Work out the finished part from the listing and answer in its coordinate system (mm). Give positions to 0.01 mm unless a question says otherwise; leave off trailing zeros. Loops run counter-clockwise (first coordinate to the right, second up) from the corner with the lowest first, then second, coordinate; pieces in that order, holes last. Notation, with made-up numbers: (31, -11) - (82, -11) arc R16 ccw to (82, -1) - close; hole circle Ø10 at (55, -8.5). An arc over 180 degrees is marked (long way). Use one line per item in the form item = value. Start each with the question number.
from build123d import *

# Parameters (mm, degrees)
BOSS_EXTRUDE1_DEPTH = 10
SKETCH2_R           = 1
CUT_EXTRUDE1_DEPTH  = 11.599213807
CHAMFER2_SIZE       = 1
FILLET1_R           = 0.5


with BuildPart() as part:
    # Sketch1 → Boss-Extrude1 (new body)
    with BuildSketch(Plane(origin=(0, 0, 0), x_dir=(1, 0, 0), z_dir=(0, 1, 0))):
        Polygon((0, 2.655811238), (-2.3, 1.327905619), (-2.3, -1.327905619), (0, -2.655811238), (2.3, -1.327905619), (2.3, 1.327905619), align=None)
    extrude(amount=BOSS_EXTRUDE1_DEPTH)

    # Sketch2 → Cut-Extrude1 (cut, through all)
    with BuildSketch(Plane(origin=(0, 10, 0), x_dir=(1, 0, 0), z_dir=(0, 1, 0))):
        with Locations(Location((0, 0, 0), (0, 0, 270))):
            Circle(SKETCH2_R)
    extrude(amount=-CUT_EXTRUDE1_DEPTH, mode=Mode.SUBTRACT)

    # Chamfer2
    chamfer2_edges = [part.edges().sort_by_distance(p)[0] for p in [
        (0, 0, -1),
        (0, 10, -1),
    ]]
    chamfer(chamfer2_edges, length=CHAMFER2_SIZE)

    # Fillet1
    fillet1_edges = [part.edges().sort_by_distance(p)[0] for p in [
        (2.3, 5, -1.327905619),
        (2.3, 5, 1.327905619),
        (0, 5, 2.655811238),
        (-2.3, 5, 1.327905619),
        (-2.3, 5, -1.327905619),
        (0, 5, -2.655811238),
    ]]
    fillet(fillet1_edges, radius=FILLET1_R)


solid = part.part
1) A cutting plane is placed at A-A (x = 0). Give the vertices of the cut face in (y, z), plus the area to 3 significant figures.
2) A cutting plane is placed at B-B (y = 6.5). Give the vertices of the cut face in (x, z), plus the area to 3 significant figures.
3) Flat-ended cylindrical pins translate along their axes: pin 1 Ø2 at (x, y) = (0.5, 8) entering from +Z; pin 2 Ø2.5 at (x, z) = (0, 0) entering from -Y. Find the tip coordinate at first contact, or state that the pin passes through.
4) Determine the mould class of faces 1 (the cylindrical face through (-1, 5, 0)), 2 (the flat face through (1.137, 4.93, 1.999)), 3 (the flat face through (2, 10, -1)) for opening direction X: released by +X, released by -X, zero draft, split by the parting line, or undercut.
5) A cutting plane is placed at D-D (z = 2.25). Give the vertices of the cut face in (x, y).
6) A cutting plane is placed at C-C (z = 0). Give the vertices of the cut face in (x, y).
7) Find the intervals of material crossed by probe 1 along X at (y, z) = (4.5, 0); probe 2 along X at (y, z) = (8, 0.85); probe 3 along Z at (x, y) = (-0.7, 7.75), in increasing order.
Answer sheet:
q1.outline = (0, -2.58) - (10, -2.58) - (10, -2) - (9, -1) - (1, -1) - (0, -2) - close; (0, 2) - (1, 1) - (9, 1) - (10, 2) - (10, 2.58) - (0, 2.58) - close
q1.area = 29.6 mm²
q2.outline = (-2.3, -1.04) arc R0.5 ccw to (-2.05, -1.47) - (-0.25, -2.51) arc R0.5 ccw to (0.25, -2.51) - (2.05, -1.47) arc R0.5 ccw to (2.3, -1.04) - (2.3, 1.04) arc R0.5 ccw to (2.05, 1.47) - (0.25, 2.51) arc R0.5 ccw to (-0.25, 2.51) - (-2.05, 1.47) arc R0.5 ccw to (-2.3, 1.04) - close; hole circle Ø2 at (0, 0)
q2.area = 15.1 mm²
q3.pin_1 = 2.58
q3.pin_2 = 0.75
q4.face_1 = undercut
q4.face_2 = released by +X
q4.face_3 = zero draft
q5.outline = (-0.7, 0) - (0.7, 0) - (0.7, 10) - (-0.7, 10) - close
q6.outline = (-2.3, 0) - (-2, 0) - (-1, 1) - (-1, 9) - (-2, 10) - (-2.3, 10) - close; (1, 1) - (2, 0) - (2.3, 0) - (2.3, 10) - (2, 10) - (1, 9) - close
q7.probe_1 = -2.3 to -1, 1 to 2.3
q7.probe_2 = -2.3 to -0.53, 0.53 to 2.3
q7.probe_3 = -2.25 to -0.71, 0.71 to 2.25
